Read the model definition and answer for the solid it produces. Units are mm, in the model's axes. Face numbers are marked on the shaded views. A direction names the side the tool comes from. Give positions to 0.01 mm unless a question says otherwise; leave off trailing zeros. Loops run counter-clockwise (first coordinate to the right, second up) from the corner with the lowest first, then second, coordinate; pieces in that order, holes last. Notation, with made-up numbers: (41, 54.25) - (80, 54.25) arc R13 ccw to (80, 69.25) - close; hole circle Ø6 at (24, -38). An arc over 180 degrees is marked (long way). Write each question's results on one line, items separated by ' | '. Start each with the question number.
Q1. Find the intervals of material crossed by line 1 (Z direction, x = 33, y = 13.5); line 2 (Y direction, x = 83.5, z = 1); line 3 (X direction, y = 78.5, z = 32), in increasing order. Write a range as from..to.
Q2. The part is cut by section B-B, the plane x = 11. Write down the section's boundary in (y, z).
Q3. The part is cut by section D-D, the plane z = 14. Write down the section's boundary in (x, y), plus the area to 3 significant figures.
Q4. The part is cut by section C-C, the plane z = -19.5. Write down the section's boundary in (x, y).
Q5. Given pin 1 (1.5 mm diameter, centred on x = -10, z = -16, fed in from +Y); pin 2 (1.5 mm diameter, centred on y = 82.5, z = 17.5, fed in from -X); pin 3 (5 mm diameter, centred on x = -52.5, y = 62, fed in from +Z), each flat-ended and moving along its own axis, determine where each tip first touches the part or whether it passes through.
Q6. The part is cut by section A-A, the plane y = 0. Write down the section's boundary in (x, z), plus the area to 3 significant figures.
Q7. For the marked faces 1, 2 and 3, determine the directions among +Z, -Z, +X, -X, +Y, -Y from which every point of the face is accessible in a straight line to the end or side of a thin tool.
```python
from build123d import *

# Parameters (mm, degrees)
SKETCH1_R           = 115
BOSS_EXTRUDE1_DEPTH = 10
SKETCH2_R           = 25
BOSS_EXTRUDE2_DEPTH = 30
SKETCH3_R           = 30
BOSS_EXTRUDE3_DEPTH = 30
CUT_EXTRUDE2_START  = -10
SKETCH4_R           = 115
SKETCH4_R_2         = 105
CUT_EXTRUDE2_DEPTH  = 10


with BuildPart() as part:
    # Sketch1 → Boss-Extrude1 (new body)
    with BuildSketch(Plane.XY):
        Circle(SKETCH1_R)
    extrude(amount=BOSS_EXTRUDE1_DEPTH)

    # Sketch2 → Boss-Extrude2 (add)
    with BuildSketch(Plane.XY.offset(10)):
        with Locations((0, 80)):
            Circle(SKETCH2_R)
    extrude(amount=BOSS_EXTRUDE2_DEPTH)

    # Sketch3 → Boss-Extrude3 (add)
    with BuildSketch(Plane(origin=(0, 0, 0), x_dir=(-1, 0, 0), z_dir=(0, 0, -1))):
        Circle(SKETCH3_R)
    extrude(amount=BOSS_EXTRUDE3_DEPTH)

    # Sketch4 → Cut-Extrude2 (cut)
    with BuildSketch(Plane.XY.offset(10).offset(CUT_EXTRUDE2_START)):
        Circle(SKETCH4_R)
        Circle(SKETCH4_R_2, mode=Mode.SUBTRACT)
    extrude(amount=CUT_EXTRUDE2_DEPTH, mode=Mode.SUBTRACT)


solid = part.part
```
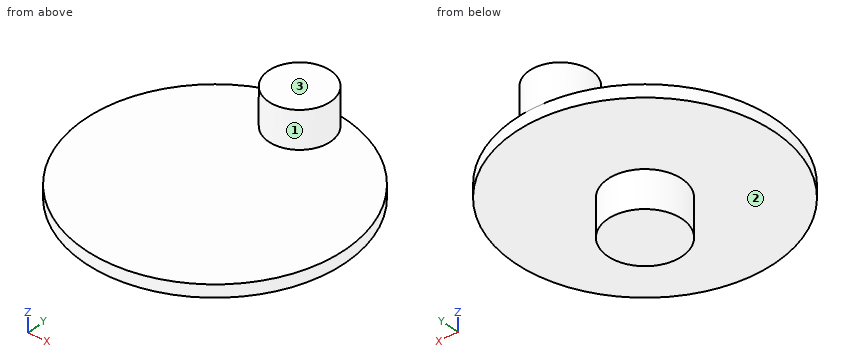
Check sheet entries:
1) line 1: z = 0..10 | line 2: y = -63.66..63.66 | line 3: x = -24.95..24.95
2) outline: (-104.42, 0) - (-27.91, 0) - (-27.91, -30) - (27.91, -30) - (27.91, 0) - (104.42, 0) - (104.42, 10) - (102.45, 10) - (102.45, 40) - (57.55, 40) - (57.55, 10) - (-104.42, 10) - close
3) outline: circle Ø50 at (0, 80) | area: 1,960 mm^2
4) outline: circle Ø60 at (0, 0)
5) pin 1: stops at y = 28.54 | pin 2: stops at x = -24.94 | pin 3: stops at z = 10
6) outline: (-105, 0) - (-30, 0) - (-30, -30) - (30, -30) - (30, 0) - (105, 0) - (105, 10) - (-105, 10) - close | area: 3,900 mm^2
7) face 1: +Z | face 2: -Z | face 3: +Z, +X, -X, +Y, -Y
